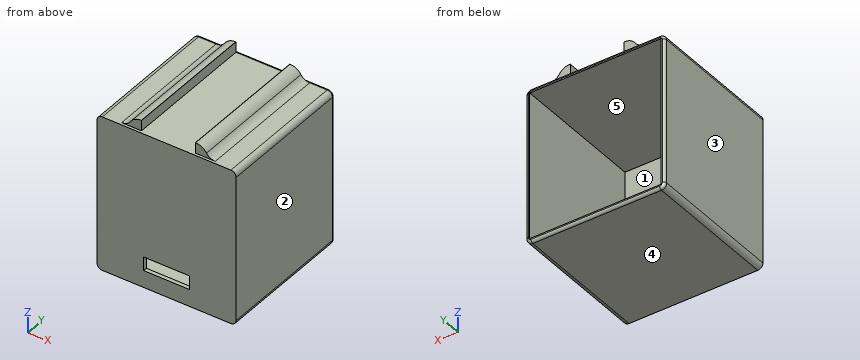
from build123d import *

# Parameters (mm, degrees)
F0_W         = 134.62
F0_H         = 134.62
F0_W_2       = 127
F0_H_2       = 127
F1_DEPTH     = 140.97
F2_W         = 134.62
F2_H         = 134.62
F3_DEPTH     = 5.08
F4_W         = 22.225
F4_H         = 13.2926666667
F5_DEPTH     = 3.81
F6_W         = 134.62
F6_H         = 134.62
F7_DEPTH     = 3.81
F8_W         = 127
F8_H         = 142.24
F9_DEPTH     = 3.81
F10_W        = 127
F10_H        = 1.27
F11_DEPTH    = 127
F12_R        = 5.08
F13_R        = 2.54
F14_W        = 12.7
F14_H        = 129.54
F15_DEPTH    = 10.16
F16_T1_DEPTH = 191.7570394667
F17_T1_DEPTH = 129.54


# Not quite as in the source:
# - a fillet or chamfer that OpenCascade refuses, or shapes differently, is made with other operations: its cross-section is extruded or revolved along the edge and cut away or added


with BuildPart() as f1:
    # F0 (on Top) → F1 (new body)
    with BuildSketch(Plane.XY):
        Rectangle(F0_W, F0_H)
        Rectangle(F0_W_2, F0_H_2, mode=Mode.SUBTRACT)
    extrude(amount=F1_DEPTH)

    # F2 (on face) → F3 (join)
    with BuildSketch(Plane.XY.offset(140.97)):
        Rectangle(F2_W, F2_H)
    extrude(amount=F3_DEPTH)

    # F4 (on face) → F5 (cut, through all)
    with BuildSketch(Plane.XZ.offset(67.31)):
        with Locations((11.1125, 19.3463333333)):
            Rectangle(F4_W, F4_H)
        with Locations((-11.1125, 19.3463333333)):
            Rectangle(F4_W, F4_H)
    extrude(amount=-F5_DEPTH, mode=Mode.SUBTRACT)

    # F6 (on face) → F7 (join)
    with BuildSketch(Plane(origin=(0, 0, 0), x_dir=(1, 0, 0), z_dir=(0, 0, -1))):
        Rectangle(F6_W, F6_H)
    extrude(amount=F7_DEPTH)

    # F8 (on face) → F9 (cut)
    with BuildSketch(Plane(origin=(0, 67.31, 0), x_dir=(-1, 0, 0), z_dir=(0, 1, 0))):
        with Locations((0, 71.12)):
            Rectangle(F8_W, F8_H)
    extrude(amount=-F9_DEPTH, mode=Mode.SUBTRACT)

    # F10 (on face) → F11 (cut, through all)
    with BuildSketch(Plane(origin=(0, 63.5, 0), x_dir=(-1, 0, 0), z_dir=(0, 1, 0))):
        with Locations((0, 141.605)):
            Rectangle(F10_W, F10_H)
    extrude(amount=-F11_DEPTH, mode=Mode.SUBTRACT)

    # F12
    f12_edges = [f1.edges().sort_by_distance(p)[0] for p in [
        (-67.31, 0, -3.81),
        (67.31, 0, -3.81),
        (67.31, 0, 146.05),
        (-67.31, 0, 146.05),
    ]]
    fillet(f12_edges, radius=F12_R)

    # F13
    f13_edges = [f1.edges().sort_by_distance(p)[0] for p in [
        (67.31, 67.31, 71.12),
        (0, 67.31, -3.81),
        (0, 67.31, 146.05),
        (-67.31, 67.31, 71.12),
        (65.822102, 67.31, 144.562102),
        (65.822102, 67.31, -2.322102),
        (-65.822102, 67.31, 144.562102),
        (-65.822102, 67.31, -2.322102),
    ]]
    fillet(f13_edges, radius=F13_R)

    # F14 (on face) → F15 (join)
    with BuildSketch(Plane.XY.offset(146.05)):
        with Locations((-32.385, 0)):
            Rectangle(F14_W, F14_H)
        with Locations((32.385, 0)):
            Rectangle(F14_W, F14_H)
    extrude(amount=F15_DEPTH)

    # F16: fillet of radius 12.7 on 2 edges, made by hand

    # F16_s2 → F16_t1 (cut)
    with BuildSketch(Plane.XZ.offset(-95.8785197333)):
        with BuildLine():
            ThreePointArc((-38.735, 146.05), (-34.3237773635, 153.3473776994), (-26.2915921067, 156.21))
            Line((-26.2915921067, 156.21), (-38.735, 156.21))
            Line((-38.735, 156.21), (-38.735, 146.05))
        make_face()
        with BuildLine():
            ThreePointArc((38.735, 146.05), (34.3237773635, 153.3473776994), (26.2915921067, 156.21))
            Line((26.2915921067, 156.21), (38.735, 156.21))
            Line((38.735, 156.21), (38.735, 146.05))
        make_face()
    extrude(amount=F16_T1_DEPTH, mode=Mode.SUBTRACT)

    # F17: fillet of radius 10.16 on 2 edges, made by hand

    # F17_s2 → F17_t1 (join)
    with BuildSketch(Plane.XZ.offset(-64.77)):
        with BuildLine():
            ThreePointArc((-36.8513807316, 150.5655555556), (-40.5097417003, 147.2497222265), (-45.2992116315, 146.05))
            Line((-45.2992116315, 146.05), (-38.735, 146.05))
            ThreePointArc((-38.735, 146.05), (-38.0126979849, 148.3993432066), (-36.8513807316, 150.5655555556))
        make_face()
        with BuildLine():
            ThreePointArc((36.8513807316, 150.5655555556), (40.5097417003, 147.2497222265), (45.2992116315, 146.05))
            Line((45.2992116315, 146.05), (38.735, 146.05))
            ThreePointArc((38.735, 146.05), (38.0126979849, 148.3993432066), (36.8513807316, 150.5655555556))
        make_face()
    extrude(amount=F17_T1_DEPTH)


solid = f1.part
The listing builds one solid part. Answer for the finished solid, in the listing's coordinates (mm). Face numbers are marked on the shaded views. A direction names the side the tool comes from. Round coordinates to 2 decimals unless told otherwise and drop trailing zeros. Order: outer loops, then holes, each group sorted by start corner. A loop starts at its lowest first (then second) coordinate and runs counter-clockwise, first axis right, second up. Notation, with made-up numbers: M 50,44 L 80,44 A28 ccw 80,81 Z; hole C 22,17 d5. An arc over 180 degrees is marked long. Answer in a Markdown table with one row per item. Add a question column.
1) The part is cut by section D-D on z = 99. Determine the outline of the cut face in (x, y).
2) The part is cut by section B-B on y = 37.5. Determine the outline of the cut face in (x, z) (3 decimals).
3) Flat-ended cylindrical pins translate along their axes: pin 1 Ø8 at (x, z) = (-32.5, 153.5) entering from +Y; pin 2 Ø12 at (x, y) = (20, -32) entering from +Z; pin 3 Ø5 at (x, z) = (38.5, 153) entering from -Y; pin 4 Ø5 at (y, z) = (30, 152.5) entering from +X. Find the tip coordinate at first contact, or state that the pin passes through.
4) Which of the six approach directions +Z, -Z, +X, -X, +Y, -Y give full straight-line access (tool end or side, diameter ignored) to the marked faces 1 and 2?
5) The part is cut by section C-C on z = 15. Determine the outline of the cut face in (x, y) (3 decimals).
6) Consider line 1 along X through (y, z) = (59, 108.5); line 2 along Z through (x, y) = (-21.5, 44.5); line 3 along Y through (x, z) = (32, 94.5). Determine where each line is inside the solid, lowest interval first. Write a range as from..to.
7) The part is cut by section A-A on x = 5.5. Determine the outline of the cut face in (y, z), plus the area to 3 significant figures.
8) Determine the mould class of the marked faces 3, 4 and 5 for opening direction Z: pulls with the +Z half, pulls with the -Z half, needs draft (parallel to the pull), parting line crosses it, or undercut.
Findings below:
| question | item | result |
|---|---|---|
| 1 | outline | M -67.31,-67.31 L 67.31,-67.31 L 67.31,64.77 A2.54 ccw 64.77,67.31 L 63.5,67.31 L 63.5,-63.5 L -63.5,-63.5 L -63.5,67.31 L -64.77,67.31 A2.54 ccw -67.31,64.77 Z |
| 2 | outline | M -67.31,1.27 A5.08 ccw -62.23,-3.81 L 62.23,-3.81 A5.08 ccw 67.31,1.27 L 67.31,140.97 A5.08 ccw 62.23,146.05 L 45.299,146.05 A10.16 cw 36.851,150.566 A12.7 ccw 26.292,156.21 L 26.035,156.21 L 26.035,146.05 L -26.035,146.05 L -26.035,156.21 L -26.292,156.21 A12.7 ccw -36.851,150.566 A10.16 cw -45.299,146.05 L -62.23,146.05 A5.08 ccw -67.31,140.97 Z; hole M -63.5,0 L 63.5,0 L 63.5,142.24 L -63.5,142.24 Z |
| 3 | pin 1 | stops at y = 64.77 |
| 3 | pin 2 | stops at z = 146.05 |
| 3 | pin 3 | passes through |
| 3 | pin 4 | stops at x = 37.26 |
| 4 | face 1 | +Y |
| 4 | face 2 | +Z, -Z, +X, +Y, -Y |
| 5 | outline | M -67.31,-67.31 L -22.225,-67.31 L -22.225,-63.5 L -63.5,-63.5 L -63.5,67.31 L -64.77,67.31 A2.54 ccw -67.31,64.77 Z; M 22.225,-67.31 L 67.31,-67.31 L 67.31,64.77 A2.54 ccw 64.77,67.31 L 63.5,67.31 L 63.5,-63.5 L 22.225,-63.5 Z |
| 6 | line 1 | x = -67.31..-63.5, 63.5..67.31 |
| 6 | line 2 | z = -3.81..0, 142.24..146.05 |
| 6 | line 3 | y = -67.31..-63.5 |
| 7 | outline | M -67.31,-3.81 L 64.77,-3.81 A2.54 ccw 67.31,-1.27 L 67.31,0 L -63.5,0 L -63.5,12.7 L -67.31,12.7 Z; M -67.31,25.99 L -63.5,25.99 L -63.5,142.24 L 67.31,142.24 L 67.31,143.51 A2.54 ccw 64.77,146.05 L -67.31,146.05 Z |
| 7 | area | 1,510 mm² |
| 8 | face 3 | needs draft |
| 8 | face 4 | pulls with the -Z half |
| 8 | face 5 | undercut |
